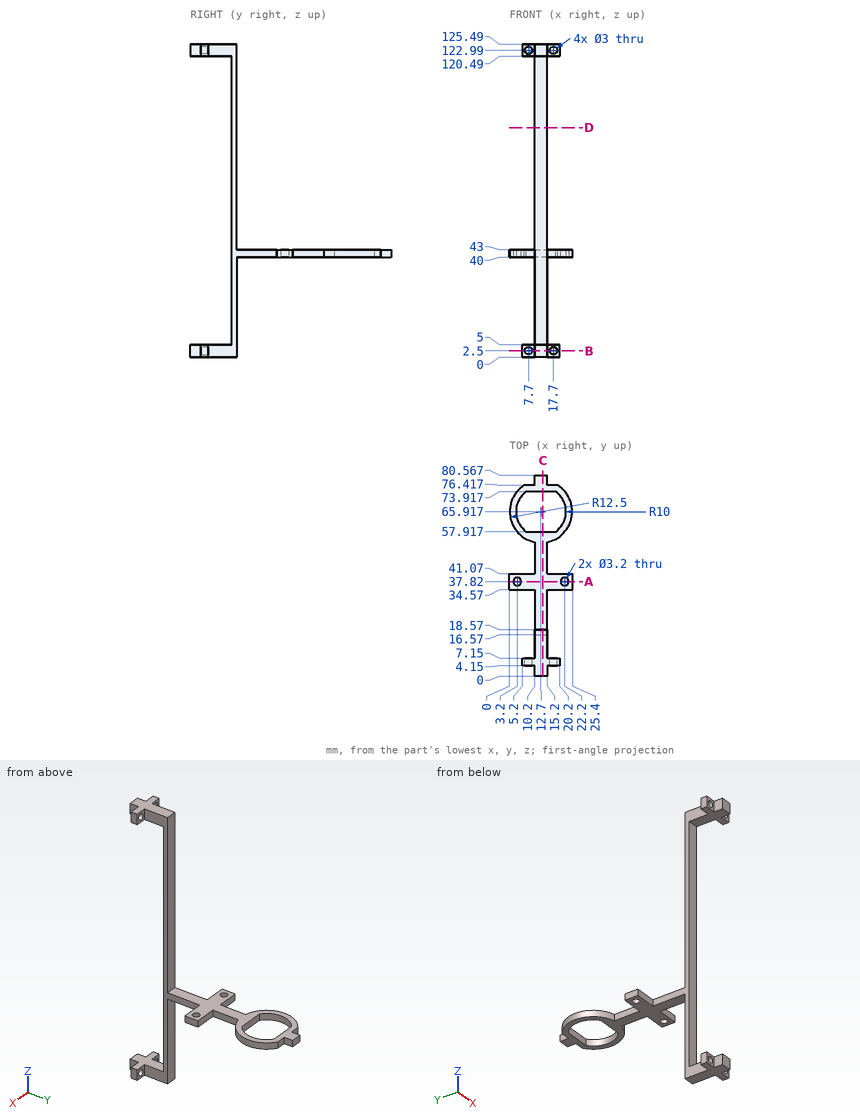
For this review, use the dimensioned drawing (mm, ordinates from the lowest corner) and the shaded views. Round coordinates to 2 decimals unless told otherwise and drop trailing zeros. Loops run counter-clockwise (first coordinate to the right, second up) from the corner with the lowest first, then second, coordinate; pieces in that order, holes last. Notation, with made-up numbers: M 52,-38.75 L 90,-38.75 A27 cw 90,-4.75 Z; hole C 64,-20 d8. An arc over 180 degrees is marked long. Answer as CSV lines item,"result".
1. We need section D-D (z = 92). Give the boundary of the cut face in (x, y), plus the area to 3 significant figures.
Outcome:
outline,"M 10.2,16.57 L 15.2,16.57 L 15.2,18.57 L 10.2,18.57 Z"
area,"10.0 mm2"
2. Insertion check: pin 1 Ø5.5 at (x, z) = (17.5, 122.5) entering from +Y; pin 2 Ø2 at (x, z) = (16, 96.5) entering from -Y; pin 3 Ø6 at (x, y) = (22.5, 33) entering from -Z; pin 4 Ø2.5 at (x, y) = (3.2, 37.82) entering from -Z. Each pin has a flat end and moves straight along its axis. Give the tip position at first contact, or say it passes through.
Outcome:
pin 1,"stops at y = 18.57"
pin 2,"stops at y = 16.57"
pin 3,"stops at z = 40"
pin 4,"passes through"
3. We need section C-C (x = 13.5). Give the boundary of the cut face in (y, z).
Outcome:
outline,"M 0,0 L 18.57,0 L 18.57,40 L 57.92,40 L 57.92,43 L 18.57,43 L 18.57,125.49 L 0,125.49 L 0,120.49 L 16.57,120.49 L 16.57,5 L 0,5 Z; M 73.92,40 L 80.57,40 L 80.57,43 L 73.92,43 Z"
4. We need section B-B (z = 2.5). Give the boundary of the cut face in (x, y).
Outcome:
outline,"M 5.2,4.15 L 6.2,4.15 L 6.2,7.15 L 5.2,7.15 Z; M 9.2,4.15 L 10.2,4.15 L 10.2,0 L 15.2,0 L 15.2,4.15 L 16.2,4.15 L 16.2,7.15 L 15.2,7.15 L 15.2,18.57 L 10.2,18.57 L 10.2,7.15 L 9.2,7.15 Z; M 19.2,4.15 L 20.2,4.15 L 20.2,7.15 L 19.2,7.15 Z"
5. To check wall thickness, follow L1, parallel to X at y = 6.5, z = 122.99; L2, parallel to Z at x = 17.7, y = 5.5; L3, parallel to Y at x = 12, z = 87. State the ranges of each line that lie inside material, in increasing order. Write a range as [from, to].
Outcome:
L1,"x = [5.2, 6.2], [9.2, 16.2], [19.2, 20.2]"
L2,"z = [0, 1], [4, 5], [120.49, 121.49], [124.49, 125.49]"
L3,"y = [16.57, 18.57]"
6. We need section A-A (y = 37.82). Give the boundary of the cut face in (x, z).
Outcome:
outline,"M 0,40 L 1.6,40 L 1.6,43 L 0,43 Z; M 4.8,40 L 20.6,40 L 20.6,43 L 4.8,43 Z; M 23.8,40 L 25.4,40 L 25.4,43 L 23.8,43 Z"
